Input: dimensioned drawing with shaded views. Units: mm. Origin: part minimum x, y, z. A direction names the side the tool comes from. Coordinates: 2 decimals unless noted, no trailing zeros. Loops run counter-clockwise (first coordinate to the right, second up) from the corner with the lowest first, then second, coordinate; pieces in that order, holes last.
Item 1: Section query A-A, the plane z = 9.74. Return the cut outline in (x, y).
Item 2: Pin query (flat end, axial travel): pin 1 Ø4 at (x, z) = (13.5, 16.5) entering from +Y; pin 2 Ø1.5 at (y, z) = (2, 2.5) entering from +X; pin 3 Ø0.9 at (x, z) = (5.5, 13.98) entering from +Y; pin 4 Ø2 at (y, z) = (2.5, 5) entering from +X. Return the tip coordinate at first contact, or that it passes through.
Item 3: Pull-direction query (X, two-part tool) for the marked faces 3, 4 and 5; classes: +X half, -X half, draft (parallel to the pull), parting line (faces both ways), or undercut.
Item 4: Reachability of the marked faces 1 and 2 from +Z, -Z, +X, -X, +Y, -Y: full face, straight path, thin tool, end or side. Return the list, or none.
Item 5: Section query B-B, the plane x = 9.74. Return the cut outline in (y, z).
Item 6: Section query D-D, the plane z = 3.74. Return the cut outline in (x, y).
Item 7: Line query: probe 1 along Z at (x, y) = (9.25, 0.85); probe 2 along X at (y, z) = (1.1, 14.5) (1 decimal); probe 3 along Y at (x, z) = (13.25, 2). Output: solid intervals per line, ascending.
Item 8: Section query C-C, the plane x = 4. Return the cut outline in (y, z).
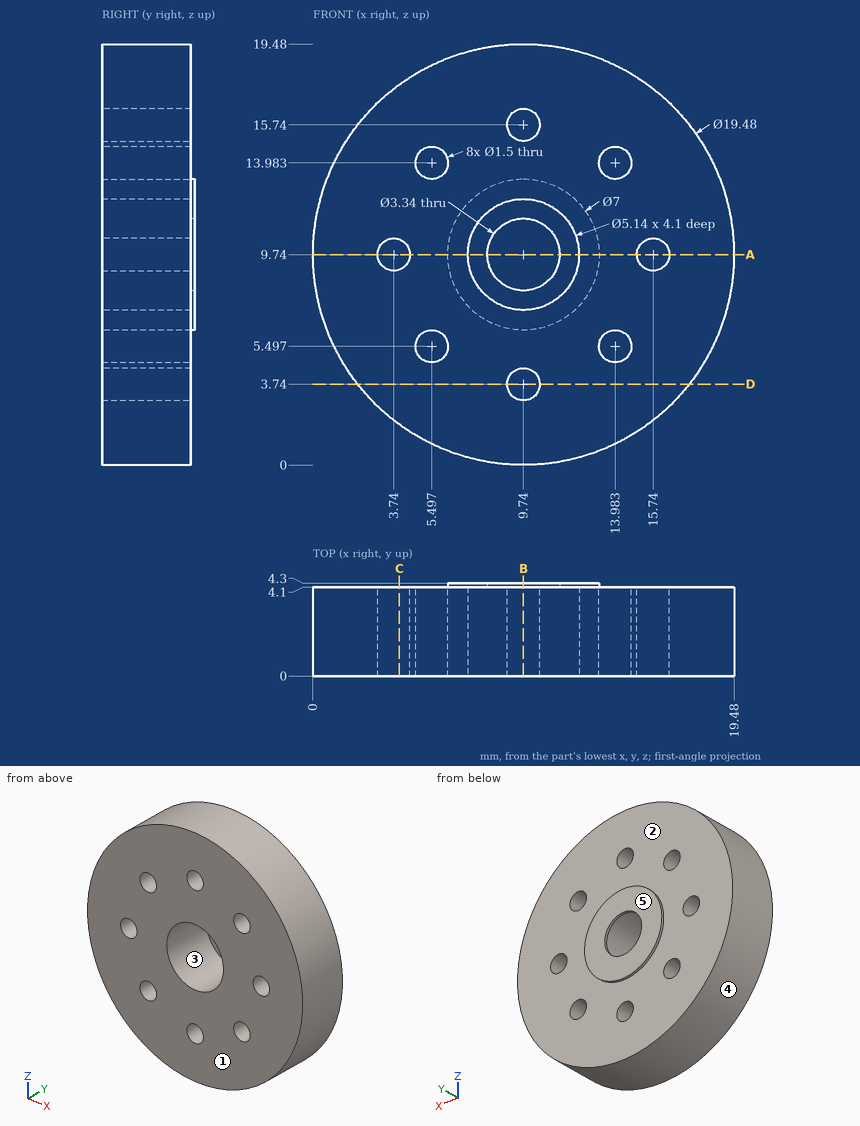
Verdict:
1. outline: (0, 0) - (2.99, 0) - (2.99, 4.1) - (0, 4.1) - close; (4.49, 0) - (7.17, 0) - (7.17, 4.1) - (8.07, 4.1) - (8.07, 4.3) - (6.24, 4.3) - (6.24, 4.1) - (4.49, 4.1) - close; (11.41, 4.1) - (12.31, 4.1) - (12.31, 0) - (14.99, 0) - (14.99, 4.1) - (13.24, 4.1) - (13.24, 4.3) - (11.41, 4.3) - close; (16.49, 0) - (19.48, 0) - (19.48, 4.1) - (16.49, 4.1) - close
2. pin 1: stops at y = 4.1
2. pin 2: stops at x = 17
2. pin 3: passes through
2. pin 4: stops at x = 18.73
3. face 3: undercut
3. face 4: parting line
3. face 5: draft
4. face 1: +Z, -Z, +X, -X, -Y
4. face 2: +Y
5. outline: (0, 0) - (4.1, 0) - (4.1, 2.99) - (0, 2.99) - close; (0, 4.49) - (4.1, 4.49) - (4.1, 6.24) - (4.3, 6.24) - (4.3, 8.07) - (4.1, 8.07) - (4.1, 7.17) - (0, 7.17) - close; (0, 12.31) - (4.1, 12.31) - (4.1, 11.41) - (4.3, 11.41) - (4.3, 13.24) - (4.1, 13.24) - (4.1, 14.99) - (0, 14.99) - close; (0, 16.49) - (4.1, 16.49) - (4.1, 19.48) - (0, 19.48) - close
6. outline: (2.07, 0) - (8.99, 0) - (8.99, 4.1) - (2.07, 4.1) - close; (10.49, 0) - (17.41, 0) - (17.41, 4.1) - (10.49, 4.1) - close
7. probe 1: z = 0.01 to 3.17, 4.31 to 7.22, 12.26 to 15.17, 16.31 to 19.47
7. probe 2: x = 1.2 to 5, 6 to 13.4, 14.5 to 18.2
7. probe 3: y = 0 to 4.1
8. outline: (0, 1.87) - (4.1, 1.87) - (4.1, 9.04) - (0, 9.04) - close; (0, 10.44) - (4.1, 10.44) - (4.1, 17.61) - (0, 17.61) - close
